The model under review builds one solid part; all positions refer to its coordinate system, in mm. A direction names the side the tool comes from. Coordinates: 2 decimals unless noted, no trailing zeros. Write each loop counter-clockwise with the first axis right and the second up, starting at its lowest first coordinate (ties: lowest second). Pieces come first, ordered by that corner, then holes.
```python
from build123d import *

# Parameters (mm, degrees)
F1_DEPTH = 30
F2_R     = 4.25
F3_DEPTH = 48.001


with BuildPart() as f1:
    # F0 (on Top) → F1 (new body)
    with BuildSketch(Plane.XY):
        with BuildLine():
            Line((35, 24), (-35, 24))
            Line((-35, 24), (-35, -24))
            Line((-35, -24), (35, -24))
            Line((35, -24), (35, -1))
            Line((35, -1), (19.974984, -1))
            ThreePointArc((19.974984, -1), (-20, 0), (19.974984, 1))
            Line((19.974984, 1), (35, 1))
            Line((35, 1), (35, 24))
        make_face()
    extrude(amount=F1_DEPTH)

    # F2 (on face) → F3 (cut, through all)
    with BuildSketch(Plane(origin=(0, 24, 0), x_dir=(-1, 0, 0), z_dir=(0, 1, 0))):
        with Locations((27, 15)):
            Circle(F2_R)
        with Locations((-27, 15)):
            Circle(F2_R)
    extrude(amount=-F3_DEPTH, mode=Mode.SUBTRACT)


solid = f1.part
```
Item 1: Take a section at A-A, the plane x = -27. Write out the cut boundary in (y, z), plus the area to 3 significant figures.
Solved:
outline: (-24, 0) - (24, 0) - (24, 10.75) - (-24, 10.75) - close; (-24, 19.25) - (24, 19.25) - (24, 30) - (-24, 30) - close
area: 1,030 mm2
Item 2: For pin 1 (7.5 mm diameter, centred on x = -27, z = 15, fed in from -Y), flat-tipped, find the tip position at first contact; note if it passes through.
Solved:
pin 1: passes through
Item 3: Mouldability with a two-part tool opening along Y and no side actions: class faces 3 (the face through (24, 1, 11)), 4 (the face through (0, -21, 30)), 5 (the face through (0, -24, 15)) as pulls with the +Y half, pulls with the -Y half, needs draft (parallel to the pull), parting line crosses it, or undercut.
Solved:
face 3: undercut
face 4: needs draft
face 5: pulls with the -Y half
Item 4: Machinability: for faces 1 (the face through (31, -1, 11)), 2 (the face through (-23.63, 0.34, 12.41)), which of the approach directions +Z, -Z, +X, -X, +Y, -Y give a long, thin tool a straight path to every point of the face, cutting with its end or side? Answer none if there is none.
Solved:
face 1: +Z, -Z, +X
face 2: +Y, -Y
Item 5: Take a section at B-B, the plane z = 15. Write out the cut boundary in (x, y), plus the area to 3 significant figures.
Solved:
outline: (-35, -24) - (-31.25, -24) - (-31.25, 24) - (-35, 24) - close; (-22.75, -24) - (22.75, -24) - (22.75, -1) - (19.97, -1) arc R20 cw (long way) to (19.97, 1) - (22.75, 1) - (22.75, 24) - (-22.75, 24) - close; (31.25, -24) - (35, -24) - (35, -1) - (31.25, -1) - close; (31.25, 1) - (35, 1) - (35, 24) - (31.25, 24) - close
area: 1,270 mm2
Item 6: To check wall thickness, follow line 1 along Z through (x, y) = (27, 9); line 2 along Y through (x, z) = (-0.5, 13.5); line 3 along Y through (x, z) = (28, 26). State the ranges of each line that lie inside material, in increasing order.
Solved:
line 1: z = 0 to 10.75, 19.25 to 30
line 2: y = -24 to -19.99, 19.99 to 24
line 3: y = -24 to -1, 1 to 24
Item 7: Take a section at D-D, the plane x = 27. Write out the cut boundary in (y, z), plus the area to 3 significant figures.
Solved:
outline: (-24, 0) - (-1, 0) - (-1, 10.75) - (-24, 10.75) - close; (-24, 19.25) - (-1, 19.25) - (-1, 30) - (-24, 30) - close; (1, 0) - (24, 0) - (24, 10.75) - (1, 10.75) - close; (1, 19.25) - (24, 19.25) - (24, 30) - (1, 30) - close
area: 989 mm2
Item 8: Take a section at C-C, the plane y = -10.5. Write out the cut boundary in (x, z), plus the area to 3 significant figures.
Solved:
outline: (-35, 0) - (-17.02, 0) - (-17.02, 30) - (-35, 30) - close; (17.02, 0) - (35, 0) - (35, 30) - (17.02, 30) - close; hole circle Ø8.5 at (-27, 15); hole circle Ø8.5 at (27, 15)
area: 965 mm2
